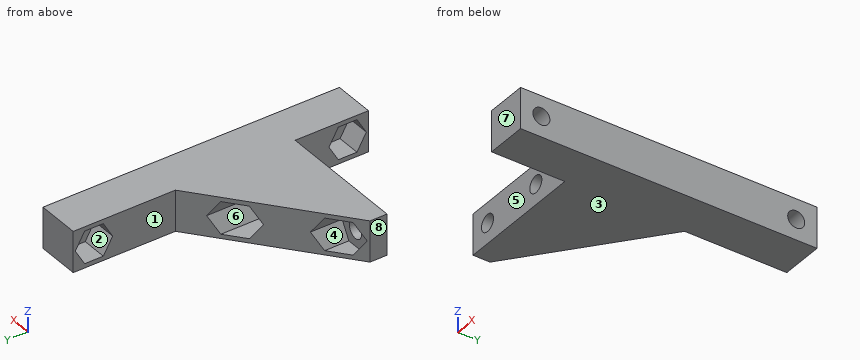
Autodesk Inventor part; units mm, degrees
ref_plane "YZ Plane" through (0, 0, 0) normal (1, 0, 0) x (0, 1, 0)
ref_plane "XZ Plane" through (0, 0, 0) normal (0, 1, 0) x (-1, 0, 0)
ref_plane "XY Plane" through (0, 0, 0) normal (0, 0, 1) x (1, 0, 0)
sketch "Sketch1" plane through (0, 0, 0) normal (0, 0, 1) x (1, 0, 0)
  line L0 (0, 0) -> (-6.096, 0)
  line L1 (-6.096, 0) -> (-6.096, 10.922)
  line L2 (-6.096, 10.922) -> (-25.4, 10.922)
  line L3 (-25.4, 10.922) -> (-25.4, 13.462)
  line L4 (-25.4, 13.462) -> (-6.35, 28.956)
  line L5 (-6.35, 28.956) -> (-6.35, 44.196)
  line L6 (-6.35, 44.196) -> (0, 44.196)
  line L7 (0, 44.196) -> (0, 0)
  dimension "d0" = 44.196
  dimension "d1" = 10.922
  dimension "d2" = 2.54
  dimension "d3" = 19.304
  dimension "d4" = 15.24
  dimension "d25" = 6.35
sketch "Sketch2" plane through (0, 0, 0) normal (1, 0, 0) x (0, 1, 0)
  line L0 (0, 3.048) -> (0, -3.048)
  line L1 (0, -3.048) -> (44.196, -3.048)
  line L2 (44.196, -3.048) -> (44.196, 3.048)
  line L3 (44.196, 3.048) -> (0, 3.048)
  circle A0 centre (3.0988, 0) radius 1.2762
  circle A1 centre (41.0972, 0) radius 1.2712
  line L4 (38.3109, 0) -> (39.7041, 2.413)
  line L5 (39.7041, 2.413) -> (42.4903, 2.413)
  line L6 (42.4903, 2.413) -> (43.8835, 0)
  line L7 (43.8835, 0) -> (42.4903, -2.413)
  line L8 (42.4903, -2.413) -> (39.7041, -2.413)
  line L9 (39.7041, -2.413) -> (38.3109, 0)
  line L10 (5.8851, -0.001) -> (4.4911, -2.4135)
  line L11 (4.4911, -2.4135) -> (1.7048, -2.4125)
  line L12 (1.7048, -2.4125) -> (0.3125, 0.001)
  line L13 (0.3125, 0.001) -> (1.7065, 2.4135)
  line L14 (1.7065, 2.4135) -> (4.4928, 2.4125)
  line L15 (4.4928, 2.4125) -> (5.8851, -0.001)
  point P0 (0, 0)
  dimension "d6" = 37.9984
  dimension "d7" = 3.0988
  dimension "d8" = 3.0988
  dimension "d9" = 44.196
  dimension "d10" = 4.826
  dimension "d11" = 6.096
  dimension "d12" = 3.048
  dimension "d13" = 4.826
sketch "Sketch3" plane through (0, 0, 0) normal (0, 1, 0) x (-1, 0, 0)
  line L0 (0, -3.048) -> (0, 3.048)
  line L1 (0, 3.048) -> (25.4, 3.048)
  line L2 (25.4, 3.048) -> (25.4, -3.048)
  line L3 (25.4, -3.048) -> (0, -3.048)
  circle A0 centre (22.352, 0) radius 1.27
  circle A1 centre (12.192, 0) radius 1.27
  line L4 (19.5657, 0) -> (20.9589, 2.413)
  line L5 (20.9589, 2.413) -> (23.7451, 2.413)
  line L6 (23.7451, 2.413) -> (25.1383, 0)
  line L7 (25.1383, 0) -> (23.7451, -2.413)
  line L8 (23.7451, -2.413) -> (20.9589, -2.413)
  line L9 (20.9589, -2.413) -> (19.5657, 0)
  line L10 (9.4057, 0) -> (10.7989, 2.413)
  line L11 (10.7989, 2.413) -> (13.5851, 2.413)
  line L12 (13.5851, 2.413) -> (14.9783, 0)
  line L13 (14.9783, 0) -> (13.5851, -2.413)
  line L14 (13.5851, -2.413) -> (10.7989, -2.413)
  line L15 (10.7989, -2.413) -> (9.4057, 0)
  point P0 (0, 0)
  dimension "d14" = 12.192
  dimension "d15" = 10.16
  dimension "d16" = 3.048
  dimension "d17" = 2.54
  dimension "d18" = 4.826
  dimension "d19" = 4.826
extrude "Extrusion1" add sketch "Sketch1" along normal mid plane 6.096
ref_plane "Work Plane1" through (-6.35, 28.956, 3.048) normal (-1, 0, 0) x (0, 0, 1)
extrude "Extrusion2" cut sketch "Sketch2" along normal blind 3.81 from surface at -6.35 contours A1 | L4 L5 L6 L7 L8 L9
extrude "Extrusion3" cut sketch "Sketch2" along normal blind 3.81 from surface at -6.35 contours A0 | L10 L11 L12 L13 L14 L15
hole "Hole1" at (0, 3.0988, 0) at (0, 41.0972, 0) direction (-1, 0, 0) diameter 2.54 end through all
ref_plane "Work Plane2" through (-25.4, 13.462, -3.048) normal (0, -1, 0) x (1, 0, 0)
extrude "Extrusion4" cut sketch "Sketch3" along normal blind 15.24 from surface at 13.462 contours A0 | A1 | L4 L5 L6 L7 L8 L9 | L10 L11 L12 L13 L14 L15
hole "Hole2" at (-22.352, 0, 0) at (-12.192, 0, 0) direction (0, 1, 0) diameter 2.54 end through all
properties part number "dispBracket"
Work out the finished part from the listing and answer in its coordinate system (mm). Face numbers are marked on the shaded views. A direction names the side the tool comes from. Round coordinates to 2 decimals unless told otherwise and drop trailing zeros. Loops run counter-clockwise (first coordinate to the right, second up) from the corner with the lowest first, then second, coordinate; pieces in that order, holes last. Notation, with made-up numbers: (-6.5, 41) - (21.5, 41) arc R18 cw to (21.5, 47) - close; hole circle Ø1 at (74, 43.25). An arc over 180 degrees is marked (long way). Use one line per item in the form item = value. Start each with the question number.
(1) Find section A-A on x = -5. Determine the outline of the cut face in (y, z).
(2) Consider line 1 (X direction, y = 12.8, z = 0); line 2 (Y direction, x = -1.9, z = 0); line 3 (Y direction, x = -6, z = 1.5). Determine where each line is inside the solid, lowest interval first.
(3) Find section D-D on y = 29.5. Determine the outline of the cut face in (x, z).
(4) Determine the mould class of the marked faces 6, 7 and 8 for opening direction X: +X half, -X half, draft (parallel to the pull), parting line (faces both ways), or undercut.
(5) Which of the six approach directions +Z, -Z, +X, -X, +Y, -Y give full straight-line access (tool end or side, diameter ignored) to the marked faces 1, 2, 3, 4 and 5?
(6) Flat-ended cylindrical pins translate along their axes: P1, Ø3, axis at x = -12.192, z = 0, coming from the -Y side; P2, Ø3.5, axis at y = 3.1, z = 0, coming from the +X side; P3, Ø1, axis at x = -12.5, z = 0, coming from the -Y side; P4, Ø1.4, axis at x = -23.5, z = -1, coming from the +Y side. Find the tip coordinate at first contact, or state that the pin passes through.
(7) Find section B-B on y = 20.5. Determine the outline of the cut face in (x, z).
(8) Find section C-C on z = 0.5. Give the number of separate pieces and of enclosed holes in the cut face, and give its area (3 significant figures).
Answer list:
q1.outline = (0, -3.05) - (44.2, -3.05) - (44.2, 3.05) - (0, 3.05) - close; hole (0.31, 0) - (1.7, -2.41) - (4.49, -2.41) - (5.89, 0) - (4.49, 2.41) - (1.71, 2.41) - close; hole (38.31, 0) - (39.7, -2.41) - (42.49, -2.41) - (43.88, 0) - (42.49, 2.41) - (39.7, 2.41) - close
q2.line_1 = -25.4 to -23.62, -21.08 to -13.46, -10.92 to 0
q2.line_2 = 0 to 1.83, 4.37 to 39.83, 42.37 to 44.2
q2.line_3 = 0 to 1.18, 5.02 to 39.18, 43.02 to 44.2
q3.outline = (-6.35, -3.05) - (0, -3.05) - (0, 3.05) - (-6.35, 3.05) - close
q4.face_6 = undercut
q4.face_7 = draft
q4.face_8 = -X half
q5.face_1 = +Z, -Z, -X, +Y
q5.face_2 = -X
q5.face_3 = -Z, +X, -X, +Y, -Y
q5.face_4 = +Y
q5.face_5 = +Z, -Z, -X, -Y
q6.P1 = 10.92
q6.P2 = 0
q6.P3 = through
q6.P4 = 13.46
q7.outline = (-16.75, -3.05) - (0, -3.05) - (0, 3.05) - (-16.75, 3.05) - close; hole (-14.98, 0) - (-13.59, -2.41) - (-10.8, -2.41) - (-9.41, 0) - (-10.8, 2.41) - (-13.59, 2.41) - close
q8.separate_pieces = 5
q8.enclosed_holes = 0
q8.area = 347 mm^2
